from build123d import *

# Parameters (mm, degrees)
SKETCH1_R                    = 2.5
BOSS_EXTRUDE1_DEPTH          = 27
CHAMFER1_SIZE                = 2
CHAMFER1_SIZE2               = 0.352653961
F_2_0_2_DIAMETER_HOLE1_D     = 2
F_2_0_2_DIAMETER_HOLE1_DEPTH = 26
F_2_0_2_DIAMETER_HOLE1_TIP   = 0.600860619
CUT_EXTRUDE1_REACH           = 29
SKETCH6_R                    = 0.25


with BuildPart() as part:
    # Sketch1 → Boss-Extrude1 (new body)
    with BuildSketch(Plane.XY):
        Circle(SKETCH1_R)
    extrude(amount=BOSS_EXTRUDE1_DEPTH)

    # Sketch3 → Cut-Revolve1 (revolve, cut)
    with BuildSketch(Plane(origin=(0, 0, 0), x_dir=(1, 0, 0), z_dir=(0, 1, 0))):
        Polygon((2.5, -11), (1.5, -13.467842271), (1.5, -17.827676266), (2.5, -19), (3.138230266, -19), (3.138230266, -11), align=None)
    revolve(axis=Axis((0, 0, 0), (0, 0, 1)), mode=Mode.SUBTRACT)

    # Chamfer1
    chamfer1_edges = [part.edges().sort_by_distance(p)[0] for p in [
        (-2.5, 0, 0),
    ]]
    chamfer1_side = [part.faces().sort_by_distance(p)[0] for p in [
        (0, 0, 0),
    ]]
    chamfer(chamfer1_edges, length=CHAMFER1_SIZE, length2=CHAMFER1_SIZE2, reference=chamfer1_side[0])

    # Ø2.0 (2) Diameter Hole1
    with Locations(Plane.XY.offset(27)):
        with Locations((0, 0)):
            Hole(F_2_0_2_DIAMETER_HOLE1_D / 2, depth=F_2_0_2_DIAMETER_HOLE1_DEPTH)
            with Locations((0, 0, -(F_2_0_2_DIAMETER_HOLE1_DEPTH + F_2_0_2_DIAMETER_HOLE1_TIP / 2))):  # 118° drill point
                Cone(0, F_2_0_2_DIAMETER_HOLE1_D / 2, F_2_0_2_DIAMETER_HOLE1_TIP, mode=Mode.SUBTRACT)

    # Sketch6 → Cut-Extrude1 (cut, up to next)
    with BuildSketch(Plane(origin=(0, 0, 0), x_dir=(-1, 0, 0), z_dir=(0, 0, -1)), mode=Mode.PRIVATE) as cut_extrude1_sk1:
        Circle(SKETCH6_R)
    cut_extrude1_tool1 = extrude(cut_extrude1_sk1.sketch, amount=-CUT_EXTRUDE1_REACH, mode=Mode.PRIVATE) & part.part
    add(cut_extrude1_tool1.solids().sort_by_distance((0, 0, 0))[0], mode=Mode.SUBTRACT)


solid = part.part
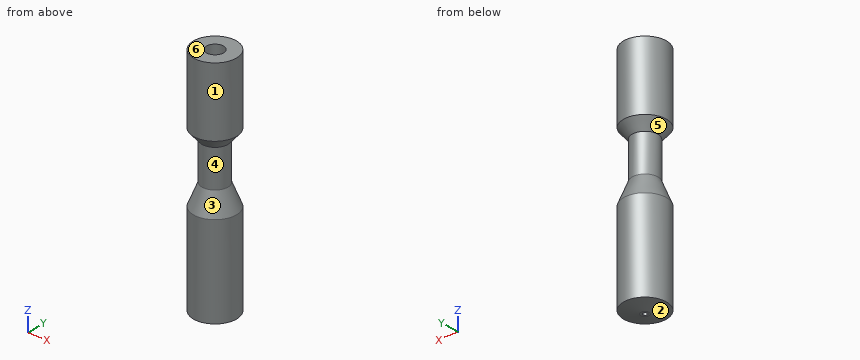
Geometry check sheet. Reference: the model listing, model coordinates, mm. Face numbers are marked on the shaded views. A direction names the side the tool comes from. Give positions to 0.01 mm unless a question says otherwise; leave off trailing zeros. Order: outer loops, then holes, each group sorted by start corner. A loop starts at its lowest first (then second) coordinate and runs counter-clockwise, first axis right, second up.
1. Sectioned sample at D-D (z = 12.25). Record the boundary of the cut face in (x, y).
Completed:
outline: circle Ø3.99 at (0, 0); hole circle Ø2 at (0, 0)
2. Sectioned sample at A-A (x = 0). Record the boundary of the cut face in (y, z).
Completed:
outline: (-2.5, 0.35) - (-0.5, 0) - (-0.25, 0) - (-0.25, 0.55) - (-1, 1) - (-1, 27) - (-2.5, 27) - (-2.5, 19) - (-1.5, 17.83) - (-1.5, 13.47) - (-2.5, 11) - close; (0.25, 0) - (0.5, 0) - (2.5, 0.35) - (2.5, 11) - (1.5, 13.47) - (1.5, 17.83) - (2.5, 19) - (2.5, 27) - (1, 27) - (1, 1) - (0.25, 0.55) - close
3. Scan lines: line 1 (Y direction, x = 0.1, z = 7.5); line 2 (Y direction, x = 0, z = 16.25); line 3 (X direction, y = -2, z = 20.75). Record each from-to range of solid material in increasing order.
Completed:
line 1: y = -2.5 to -0.99, 0.99 to 2.5
line 2: y = -1.5 to -1, 1 to 1.5
line 3: x = -1.5 to 1.5
4. Access from +Z, -Z, +X, -X, +Y, -Y to the whole of each face (thin tool, end or side, straight path). Record for the marked faces 5 and 6.
Completed:
face 5: none
face 6: +Z, +X, -X, +Y, -Y
5. Sectioned sample at C-C (z = 6). Record the boundary of the cut face in (x, y).
Completed:
outline: circle Ø5 at (0, 0); hole circle Ø2 at (0, 0)
6. Draft check along Z on the marked faces 1, 2, 3 and 4. Enter one of: pulls with the +Z half, pulls with the -Z half, needs draft (parallel to the pull), parting line crosses it, or undercut.
Completed:
face 1: needs draft
face 2: pulls with the -Z half
face 3: undercut
face 4: undercut
7. Depth check by flat-ended pin: pin 1 (1.5 mm diameter, centred on x = 1.5, z = 17, fed in from -Y); pin 2 (3 mm diameter, centred on y = 1.5, z = 14.5, fed in from +X); pin 3 (3 mm diameter, centred on x = 0, y = 0, fed in from -Z). Enter the tip coordinate at first touch or a pass-through.
Completed:
pin 1: stops at y = -1.3
pin 2: stops at x = 1.5
pin 3: stops at z = 0
